Work out the finished part from the listing and answer in its coordinate system (mm). A direction names the side the tool comes from. Round coordinates to 2 decimals unless told otherwise and drop trailing zeros. Write each loop counter-clockwise with the first axis right and the second up, starting at its lowest first coordinate (ties: lowest second). Pieces come first, ordered by that corner, then holes. Notation, with made-up numbers: (81.25, 1) -> (136.25, 1) arc R21 ccw to (136.25, 25) -> close; hole circle Ø6 at (-7, 5). An arc over 180 degrees is marked (long way). One line per item, written item: value.
```python
from build123d import *

# Parameters (mm, degrees)
SKETCH_1_W          = 50
SKETCH_1_H          = 20
EXTRUDE_1_DEPTH     = 3
SKETCH_2_W          = 50
SKETCH_2_H          = 15
EXTRUDE_2_DEPTH     = 6
SKETCH_5_W          = 50
SKETCH_5_H          = 12
CUT_EXTRUDE_2_DEPTH = 3
SKETCH_7_R          = 1.65
EXTRUDE_3_DEPTH     = 3
SKETCH_8_R          = 1.65
CUT_EXTRUDE_3_DEPTH = 3


with BuildPart() as part:
    # 草图1 → 凸台-拉伸1 (new body)
    with BuildSketch(Plane.XY):
        Rectangle(SKETCH_1_W, SKETCH_1_H)
        with BuildLine():
            Line((-4.708438024, 2.5), (4.708438024, 2.5))
            ThreePointArc((4.708438024, 2.5), (5.261208823, 2.666666667), (5.629722688, 3.111111111))
            ThreePointArc((5.629722688, 3.111111111), (21, 0), (5.629722688, -3.111111111))
            ThreePointArc((5.629722688, -3.111111111), (5.261208823, -2.666666667), (4.708438024, -2.5))
            Line((4.708438024, -2.5), (-4.708438024, -2.5))
            ThreePointArc((-4.708438024, -2.5), (-5.261208823, -2.666666667), (-5.629722688, -3.111111111))
            ThreePointArc((-5.629722688, -3.111111111), (-21, 0), (-5.629722688, 3.111111111))
            ThreePointArc((-5.629722688, 3.111111111), (-5.261208823, 2.666666667), (-4.708438024, 2.5))
        make_face(mode=Mode.SUBTRACT)
        with BuildLine():
            Line((3.25, 5.5), (-3.25, 5.5))
            ThreePointArc((-3.25, 5.5), (-5, 7.25), (-3.25, 9))
            Line((-3.25, 9), (3.25, 9))
            ThreePointArc((3.25, 9), (5, 7.25), (3.25, 5.5))
        make_face(mode=Mode.SUBTRACT)
    extrude(amount=EXTRUDE_1_DEPTH)

    # 草图2 → 凸台-拉伸2 (add)
    with BuildSketch(Plane(origin=(0, 10, 0), x_dir=(1, 0, 0), z_dir=(0, 1, 0))):
        with Locations((0, -7.5)):
            Rectangle(SKETCH_2_W, SKETCH_2_H)
    extrude(amount=EXTRUDE_2_DEPTH)

    # 草图5 → 切除-拉伸2 (cut)
    with BuildSketch(Plane.XZ.offset(-10)):
        with Locations((0, 9)):
            Rectangle(SKETCH_5_W, SKETCH_5_H)
    extrude(amount=-CUT_EXTRUDE_2_DEPTH, mode=Mode.SUBTRACT)

    # 草图7 → 凸台-拉伸3 (add)
    with BuildSketch(Plane(origin=(0, 16, 0), x_dir=(1, 0, 0), z_dir=(0, 1, 0))):
        Polygon((-0.251262658, -31.819805153), (-17.071067812, -15), (16.568542495, -15), align=None)
        with Locations(Location((-0.251262658, -24.748737342, 0), (0, 0, 180))):
            Circle(SKETCH_7_R, mode=Mode.SUBTRACT)
    extrude(amount=-EXTRUDE_3_DEPTH)

    # 草图8 → 切除-拉伸3 (cut)
    with BuildSketch(Plane(origin=(0, 16, 0), x_dir=(1, 0, 0), z_dir=(0, 1, 0))):
        with Locations(Location((-16.514718626, -8.485281374, 0), (0, 0, 180))):
            Circle(SKETCH_8_R)
    extrude(amount=-CUT_EXTRUDE_3_DEPTH, mode=Mode.SUBTRACT)


solid = part.part
```
(1) For a pull along X with two mould halves and no side action, classify faces 4 (the face through (0, -10, 1)), 5 (the face through (8.28, 14.52, 23.29)), 6 (the face through (5, 7.3, 1.5)) as pulls with the +X half, pulls with the -X half, needs draft (parallel to the pull), parting line crosses it, or undercut.
Reported:
face 4: needs draft
face 5: pulls with the +X half
face 6: undercut
(2) Find section B-B on x = 14. Give the vertices of the cut face in (y, z), plus the area to 3 significant figures.
Reported:
outline: (-10, 0) -> (-7.94, 0) -> (-7.94, 3) -> (-10, 3) -> close; (7.94, 0) -> (16, 0) -> (16, 17.57) -> (13, 17.57) -> (13, 3) -> (7.94, 3) -> close
area: 74.1 mm2
(3) Find section D-D on z = 13.5. Give the vertices of the cut face in (x, y).
Reported:
outline: (-25, 13) -> (25, 13) -> (25, 16) -> (-25, 16) -> close
(4) Find section A-A on y = 0. Give the vertices of the cut face in (x, z), plus the area to 3 significant figures.
Reported:
outline: (-25, 0) -> (-21, 0) -> (-21, 3) -> (-25, 3) -> close; (21, 0) -> (25, 0) -> (25, 3) -> (21, 3) -> close
area: 24.0 mm2
(5) Consider probe 1 along X at (y, z) = (0, 2); probe 2 along Y at (x, z) = (-13, 2.2); probe 3 along Z at (x, y) = (-16, -8.5). Determine where each line is inside the solid, lowest interval first.
Reported:
probe 1: x = -25 to -21, 21 to 25
probe 2: y = -10 to -8, 8 to 16
probe 3: z = 0 to 3
(6) Find section C-C on y = 7.25. Give the vertices of the cut face in (x, z).
Reported:
outline: (-25, 0) -> (-16.38, 0) -> (-16.38, 3) -> (-25, 3) -> close; (-9.62, 0) -> (-5, 0) -> (-5, 3) -> (-9.62, 3) -> close; (5, 0) -> (9.62, 0) -> (9.62, 3) -> (5, 3) -> close; (16.38, 0) -> (25, 0) -> (25, 3) -> (16.38, 3) -> close
(7) Flat-ended cylindrical pins translate along their axes: pin 1 Ø4 at (x, z) = (-5, 19) entering from -Y; pin 2 Ø5 at (x, y) = (-2.5, 4.5) entering from +Z; pin 3 Ø2.5 at (x, y) = (21.5, 15) entering from +Z; pin 4 Ø1.5 at (x, y) = (7.5, 1.5) entering from +Z. Find the tip coordinate at first contact, or state that the pin passes through.
Reported:
pin 1: stops at y = 13
pin 2: stops at z = 3
pin 3: stops at z = 15
pin 4: passes through
(8) A tool of negligible diameter and unlimited length cuts with its end or side. For faces 1 (the face through (21, 14, 15)), 2 (the face through (0, 5.5, 1)), 3 (the face through (0, 4, 3)), from which of +Z, -Z, +X, -X, +Y, -Y can it reach the whole face along a straight path? Write none if from no direction.
Reported:
face 1: +Z, +X, +Y, -Y
face 2: +Z, -Z
face 3: +Z, +X, -X, -Y
